from build123d import *

# Parameters (mm, degrees)
EXTRUDE_1_DEPTH          = 5
SKETCH_3_R               = 5
EXTRUDE_2_DEPTH          = 17
SKETCH_4_R               = 3
CUT_EXTRUDE_1_DEPTH      = 17
SKETCH_6_R               = 1.5
CUT_EXTRUDE_2_DEPTH      = 5
CUT_EXTRUDE_2_DEPTH_BACK = 5


with BuildPart() as part:
    # 草图1 → 凸台-拉伸1 (new body)
    with BuildSketch(Plane(origin=(0, 0, 0), x_dir=(1, 0, 0), z_dir=(0, 1, 0))):
        Polygon((-7, 0), (-3.5, -6.062177826), (3.5, -6.062177826), (7, 0), (3.5, 6.062177826), (-3.5, 6.062177826), align=None)
    extrude(amount=EXTRUDE_1_DEPTH)

    # 草图3 → 凸台-拉伸2 (add)
    with BuildSketch(Plane(origin=(0, 0, 0), x_dir=(1, 0, 0), z_dir=(0, 1, 0))):
        Circle(SKETCH_3_R)
    extrude(amount=EXTRUDE_2_DEPTH)

    # 草图4 → 切除-拉伸1 (cut)
    with BuildSketch(Plane(origin=(0, 0, 0), x_dir=(1, 0, 0), z_dir=(0, 1, 0))):
        Circle(SKETCH_4_R)
    extrude(amount=CUT_EXTRUDE_1_DEPTH, mode=Mode.SUBTRACT)

    # 草图6 → 切除-拉伸2 (cut, two sides)
    with BuildSketch(Plane.XY) as cut_extrude_2_sk:
        with Locations((0, 13.047463788)):
            Circle(SKETCH_6_R)
    extrude(amount=CUT_EXTRUDE_2_DEPTH, mode=Mode.SUBTRACT)
    extrude(cut_extrude_2_sk.sketch, amount=-CUT_EXTRUDE_2_DEPTH_BACK, mode=Mode.SUBTRACT)


solid = part.part
Geometry: final body of the model. Coordinates: model frame, mm. A direction names the side the tool comes from. Give positions to 0.01 mm unless a question says otherwise; leave off trailing zeros. Order: outer loops, then holes, each group sorted by start corner. A loop starts at its lowest first (then second) coordinate and runs counter-clockwise, first axis right, second up. Notation, with made-up numbers: (68, 46) -> (87, 46) arc R21 cw to (87, 65) -> close; hole circle Ø7 at (83, 75.25). An arc over 180 degrees is marked (long way). Answer as a JSON object with one key per item and string values.
Q1. First-contact query: pin 1 (1.5 mm diameter, centred on x = -1, z = 2.5, fed in from -Y); pin 2 (5 mm diameter, centred on x = 0, y = 13.05, fed in from -Z); pin 3 (3 mm diameter, centred on y = 11.5, z = 1, fed in from -X). Flat tips, straight axial feed; report the tip coordinate or a pass-through.
Entries:
{"pin 1": "stops at y = 0", "pin 2": "stops at z = -5", "pin 3": "stops at x = -5"}
Q2. Access query for faces 1 (the flat face through (5.274, 2.465, -2.989)), 2 (the cylindrical face through (4.619, 10.916, 1.915)). Directions: +Z, -Z, +X, -X, +Y, -Y. A direction counts if a zero-diameter tool reaches every point of the face in a straight line with its end or side. Return the directions, or none.
Entries:
{"face 1": "-Z, +X, +Y, -Y", "face 2": "+Y"}
Q3. Section A-A (x = 0). Output: boundary loops of the cut face in (y, z), plus the area to 3 significant figures.
Entries:
{"outline": "(0, -6.06) -> (5, -6.06) -> (5, -5) -> (11.55, -5) -> (11.55, -3) -> (0, -3) -> close; (0, 3) -> (11.55, 3) -> (11.55, 5) -> (5, 5) -> (5, 6.06) -> (0, 6.06) -> close; (14.55, -5) -> (17, -5) -> (17, -3) -> (14.55, -3) -> close; (14.55, 3) -> (17, 3) -> (17, 5) -> (14.55, 5) -> close", "area": "66.6 mm^2"}
Q4. Section D-D (y = 6.25). Output: boundary loops of the cut face in (x, z).
Entries:
{"outline": "circle Ø10 at (0, 0); hole circle Ø6 at (0, 0)"}
Q5. Section B-B (z = 1.5). Output: boundary loops of the cut face in (x, y).
Entries:
{"outline": "(-6.13, 0) -> (-2.6, 0) -> (-2.6, 17) -> (-4.77, 17) -> (-4.77, 5) -> (-6.13, 5) -> close; (2.6, 0) -> (6.13, 0) -> (6.13, 5) -> (4.77, 5) -> (4.77, 17) -> (2.6, 17) -> close"}
Q6. Material intervals for probe 1 along Z at (x, y) = (0, 11); probe 2 along Y at (x, z) = (0, 3.3); probe 3 along Y at (x, z) = (-3.25, 5.25), sorted ascending.
Entries:
{"probe 1": "z = -5 to -3, 3 to 5", "probe 2": "y = 0 to 11.55, 14.55 to 17", "probe 3": "y = 0 to 5"}
Q7. Section C-C (y = 14.25). Output: boundary loops of the cut face in (x, z), plus the area to 3 significant figures.
Entries:
{"outline": "(-0.9, -4.92) -> (-0.9, -2.86) arc R3 cw to (-0.9, 2.86) -> (-0.9, 4.92) arc R5 ccw to start; (0.9, -4.92) arc R5 ccw to (0.9, 4.92) -> (0.9, 2.86) arc R3 cw to (0.9, -2.86) -> close", "area": "43.0 mm^2"}
Q8. Draft query along X for faces 3 (the flat face through (5.226, 2.465, 3.074)), 4 (the cylindrical face through (1.386, 12.473, 3.783)), 5 (the flat face through (-5.226, 2.465, -3.074)), 6 (the flat face through (0, 2, -6.062)). Return one class per face: released by +X, released by -X, zero draft, split by the parting line, or undercut.
Entries:
{"face 3": "released by +X", "face 4": "undercut", "face 5": "released by -X", "face 6": "zero draft"}
